Work out the finished part from the listing and answer in its coordinate system (mm). Face numbers are marked on the shaded views. Round coordinates to 2 decimals unless told otherwise and drop trailing zeros. Write each loop counter-clockwise with the first axis right and the second up, starting at its lowest first coordinate (ties: lowest second). Pieces come first, ordered by that corner, then holes.
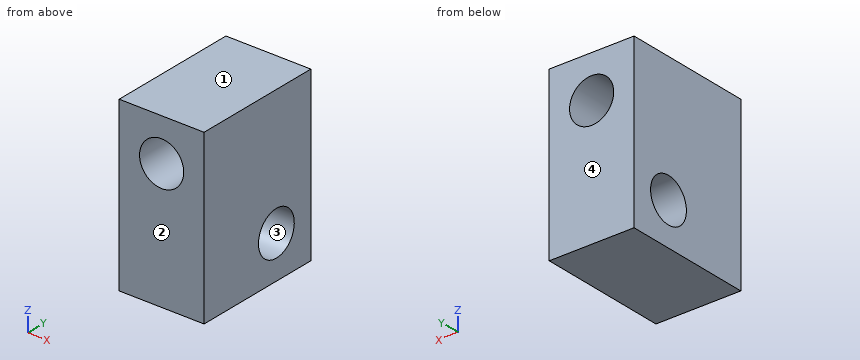
Autodesk Inventor part; units mm, degrees
ref_plane "YZ Plane" through (0, 0, 0) normal (1, 0, 0) x (0, 1, 0)
ref_plane "XZ Plane" through (0, 0, 0) normal (0, 1, 0) x (-1, 0, 0)
ref_plane "XY Plane" through (0, 0, 0) normal (0, 0, 1) x (1, 0, 0)
sketch "Sketch1" plane through (0, 0, 0) normal (0, 1, 0) x (-1, 0, 0)
  line L0 (0, 0) -> (0, -5.5)
  line L1 (0, -5.5) -> (0, -15.5)
  circle A0 centre (0, -15.5) radius 2.6
  line L2 (0, -100) -> (0, -84.8)
  circle A1 centre (0, -84.8) radius 2.6
  line L3 (0, -50) -> (0, -26)
  line L4 (0, -26) -> (-5, -26)
  line L5 (0, -12.9) -> (0, -10.5)
  line L6 (0, -10.5) -> (-5, -10.5)
  line L7 (-5, -10.5) -> (-5, -26)
  line L8 (0, -10.5) -> (5, -10.5)
  line L9 (5, -10.5) -> (5, -26)
  line L10 (5, -26) -> (0, -26)
  line L11 (0, 0) -> (0, -12.9)
  line L12 (0, -18.1) -> (0, -100)
  line L13 (0, 0) -> (5, 0)
  line L14 (0, 0) -> (-5, 0)
  line L15 (0, 0) -> (0, 5)
  line L16 (0, 5) -> (0, 12.4)
  line L17 (0, 15) -> (0, 20)
  line L18 (0, 20) -> (-5, 20)
  line L19 (-5, 20) -> (-5, 0)
  line L20 (5, 0) -> (5, 20)
  line L21 (5, 20) -> (0, 20)
  circle A2 centre (0, 15) radius 2.6
  dimension "d15" = 5.2
  dimension "d0" = 100
  dimension "d1" = 5.5
  dimension "d2" = 10
  dimension "d3" = 5.2
  dimension "d4" = 15.2
  dimension "d5" = 5.2
  dimension "d6" = 24
  dimension "d7" = 5
  dimension "d8" = 5
  dimension "d9" = 5
  dimension "d10" = 5
  dimension "d11" = 5
  dimension "d12" = 5
  dimension "d13" = 10
  dimension "d14" = 5
extrude "Extrusion1" add sketch "Sketch1" along normal blind 15.5 contours L15 L16 A2 L17 L21 L20 L13 | L14 L19 L18 L17 A2 L16 L15
sketch "Sketch2" plane through (5, 0, 20) normal (1, 0, 0) x (0, 0, -1)
  line L0 (20, 15.5) -> (15, 15.5)
  line L1 (20, 15.5) -> (0, 15.5)
  line L2 (15, 15.5) -> (15, 10.5)
  circle A0 centre (15, 10.5) radius 2.6
  point P0 (20, 0)
  dimension "d18" = 5
  dimension "d19" = 5
  dimension "d20" = 5.2
extrude "Extrusion2" cut sketch "Sketch2" against normal blind 15.5
properties part number "roller_joint_front"
Q1. The mould has two halves that part along Y. Classify the marked faces 1, 2, 3 and 4: +Y half, -Y half, draft (parallel to the pull), parting line (faces both ways), or undercut.
Q2. Find section B-B (x = 0). Determine the outline of the cut face in (y, z), plus the area to 3 significant figures.
Q3. Find section D-D (z = 5). Determine the outline of the cut face in (x, y).
Q4. Find the intervals of material crossed by L1, parallel to X at y = 10, z = 15; L2, parallel to Y at x = -3, z = 5; L3, parallel to Z at x = 2.75, y = 10.5, in increasing order.
Q5. Find section A-A (y = 11.5). Determine the outline of the cut face in (x, z), plus the area to 3 significant figures.
Q6. Find section C-C (z = 15). Determine the outline of the cut face in (x, y), plus the area to 3 significant figures.
Report:
1. face 1: draft
1. face 2: -Y half
1. face 3: undercut
1. face 4: +Y half
2. outline: (0, 0) - (15.5, 0) - (15.5, 12.4) - (0, 12.4) - close; (0, 17.6) - (15.5, 17.6) - (15.5, 20) - (0, 20) - close; hole circle Ø5.2 at (10.5, 5)
2. area: 208 mm2
3. outline: (-5, 0) - (5, 0) - (5, 7.9) - (-5, 7.9) - close; (-5, 13.1) - (5, 13.1) - (5, 15.5) - (-5, 15.5) - close
4. L1: x = -5 to -2.6, 2.6 to 5
4. L2: y = 0 to 7.9, 13.1 to 15.5
4. L3: z = 0 to 2.4, 7.6 to 20
5. outline: (-5, 0) - (5, 0) - (5, 2.6) - (-5, 2.6) - close; (-5, 7.4) - (5, 7.4) - (5, 20) - (-5, 20) - close; hole circle Ø5.2 at (0, 15)
5. area: 131 mm2
6. outline: (-5, 0) - (-2.6, 0) - (-2.6, 15.5) - (-5, 15.5) - close; (2.6, 0) - (5, 0) - (5, 15.5) - (2.6, 15.5) - close
6. area: 74.4 mm2
